Study the drawing (mm; zero at the part's minimum x, y, z) and answer. A direction names the side the tool comes from. Give positions to 0.01 mm unless a question says otherwise; leave off trailing zeros. Write each loop counter-clockwise with the first axis right and the second up, starting at its lowest first coordinate (ties: lowest second). Pieces come first, ordered by that corner, then holes. Notation, with made-up numbers: (49.25, -34.75) - (94.25, -34.75) arc R10 ccw to (94.25, -23.75) - close; hole circle Ø7 at (-2, 76). An arc over 180 degrees is marked (long way). Return JSON: item names as keys, results as strings.
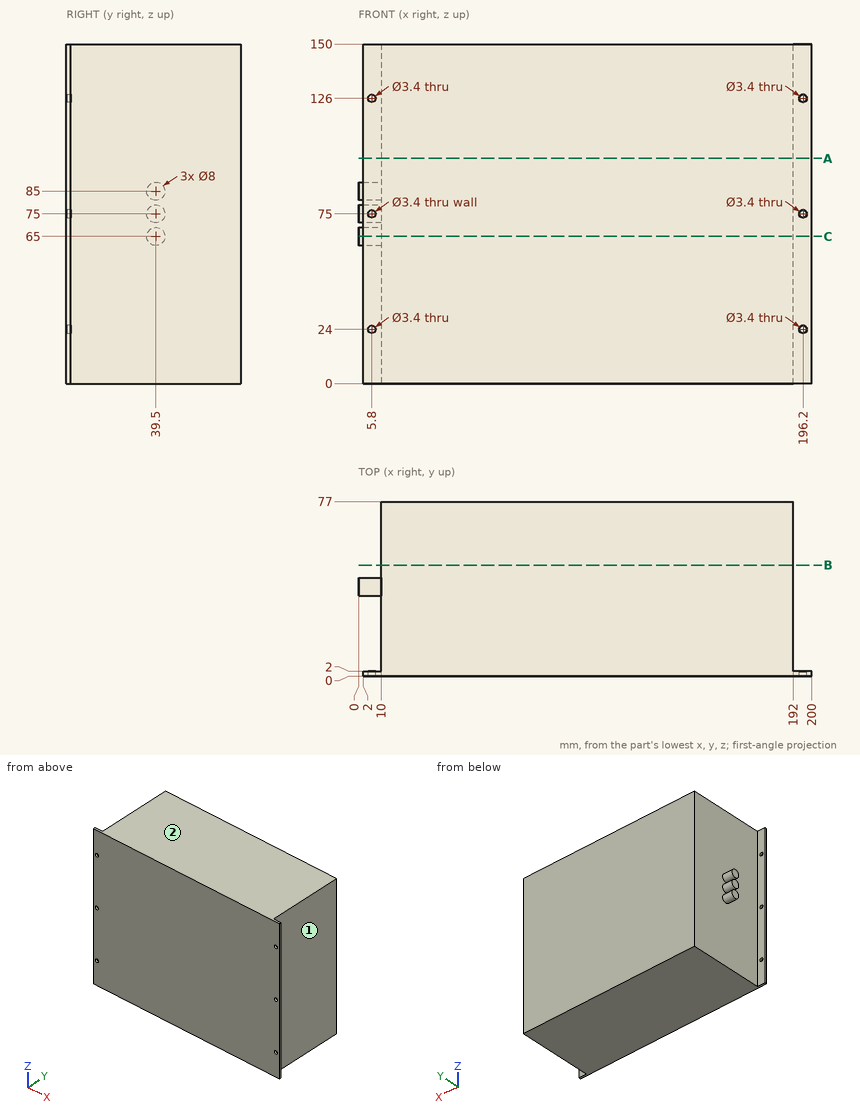
Item 1: A cutting plane is placed at B-B on y = 49. Determine the outline of the cut face in (x, z), then the cut area to 3 significant figures.
Answer below:
{"outline": "(10, 0) - (192, 0) - (192, 150) - (10, 150) - close", "area": "27,300 mm²"}
Item 2: A cutting plane is placed at C-C on z = 65. Determine the outline of the cut face in (x, y), then the cut area to 3 significant figures.
Answer below:
{"outline": "(0, 35.5) - (10, 35.5) - (10, 2) - (2, 2) - (2, 0) - (200, 0) - (200, 2) - (192, 2) - (192, 77) - (10, 77) - (10, 43.5) - (0, 43.5) - close", "area": "14,100 mm²"}
Item 3: Consider L1, parallel to Z at x = 196.2, y = 1.1; L2, parallel to X at y = 0.9, z = 75; L3, parallel to Z at x = 5, y = 1. Determine where each line is inside the solid, lowest interval first.
Answer below:
{"L1": "z = 0 to 22.3, 25.7 to 73.3, 76.7 to 124.3, 127.7 to 150", "L2": "x = 2 to 4.1, 7.5 to 194.5, 197.9 to 200", "L3": "z = 0 to 22.5, 25.5 to 73.5, 76.5 to 124.5, 127.5 to 150"}
Item 4: Flat-ended cylindrical pins translate along their axes: P1, Ø12, axis at y = 32.5, z = 95, coming from the -X side; P2, Ø1, axis at y = 0.5, z = 48.5, coming from the -X side; P3, Ø4.5, axis at x = 196.2, z = 24, coming from the +Y side. Find the tip coordinate at first contact, or state that the pin passes through.
Answer below:
{"P1": "stops at x = 10", "P2": "stops at x = 2", "P3": "stops at y = 2"}
Item 5: A cutting plane is placed at A-A on z = 99.5. Determine the outline of the cut face in (x, y).
Answer below:
{"outline": "(2, 0) - (200, 0) - (200, 2) - (192, 2) - (192, 77) - (10, 77) - (10, 2) - (2, 2) - close"}
Item 6: For the marked faces 1 and 2, determine the directions among +Z, -Z, +X, -X, +Y, -Y from which every point of the face is accessible in a straight line to the end or side of a thin tool.
Answer below:
{"face 1": "+Z, -Z, +X, +Y", "face 2": "+Z, +X, -X, +Y, -Y"}
